from build123d import *

# Parameters (mm, degrees)
SKETCH_1_W          = 6
SKETCH_1_H          = 6
EXTRUDE_1_DEPTH     = 27
SKETCH_2_W          = 2
SKETCH_2_H          = 3
EXTRUDE_2_DEPTH     = 6
SKETCH_3_R          = 0.75
EXTRUDE_3_DEPTH     = 1
SKETCH_5_W          = 18
SKETCH_5_H          = 3.5
CUT_EXTRUDE_1_DEPTH = 8
SKETCH_6_R          = 1.5
CUT_EXTRUDE_2_DEPTH = 8
SKETCH_7_R          = 0.9
CUT_EXTRUDE_3_DEPTH = 8


with BuildPart() as part:
    # 草图1 → 凸台-拉伸1 (new body)
    with BuildSketch(Plane.XY):
        Rectangle(SKETCH_1_W, SKETCH_1_H)
    extrude(amount=EXTRUDE_1_DEPTH)

    # 草图2 → 凸台-拉伸2 (add)
    with BuildSketch(Plane.XY.offset(27)):
        with Locations((-1.14479355, -0.004540815)):
            Rectangle(SKETCH_2_W, SKETCH_2_H)
    extrude(amount=EXTRUDE_2_DEPTH)

    # 草图3 → 凸台-拉伸3 (add)
    with BuildSketch(Plane.ZY.offset(2.14479355)):
        with Locations(Location((31, 0, 0), (0, 0, 90))):
            Circle(SKETCH_3_R)
    extrude(amount=EXTRUDE_3_DEPTH)

    # 草图4 → 旋转1 (revolve)
    with BuildSketch(Plane(origin=(0, 0, 0), x_dir=(1, 0, 0), z_dir=(0, 1, 0))):
        with BuildLine():
            Line((-3.14479355, -31), (-6.998843172, -31))
            ThreePointArc((-6.998843172, -31), (-5.380877697, -29.036826645), (-3.14479355, -30.25))
            Line((-3.14479355, -30.25), (-3.14479355, -31))
        make_face()
    revolve(axis=Axis((-3.14479355, 0, 31), (-1, 0, 0)))

    # 草图5 → 切除-拉伸1 (cut)
    with BuildSketch(Plane(origin=(0.5, 3, 0), x_dir=(0, 0, 1), z_dir=(0, -1, 0))):
        with Locations((13.5, 0.5)):
            Rectangle(SKETCH_5_W, SKETCH_5_H)
    extrude(amount=CUT_EXTRUDE_1_DEPTH, mode=Mode.SUBTRACT)

    # 草图6 → 切除-拉伸2 (cut)
    with BuildSketch(Plane.ZY.offset(3)):
        with Locations((16, 0)):
            Circle(SKETCH_6_R)
    extrude(amount=-CUT_EXTRUDE_2_DEPTH, mode=Mode.SUBTRACT)

    # 草图7 → 切除-拉伸3 (cut)
    with BuildSketch(Plane(origin=(0, 0, 0), x_dir=(-1, 0, 0), z_dir=(0, 0, -1))):
        Circle(SKETCH_7_R)
    extrude(amount=-CUT_EXTRUDE_3_DEPTH, mode=Mode.SUBTRACT)


solid = part.part
Part model, mm, in its own coordinate system. A direction names the side the tool comes from. Coordinates: 2 decimals unless noted, no trailing zeros. Loops run counter-clockwise (first coordinate to the right, second up) from the corner with the lowest first, then second, coordinate; pieces in that order, holes last. Notation, with made-up numbers: M 37,-32.75 L 71,-32.75 A16 cw 71,-8.75 Z; hole C 64,80 d3. An arc over 180 degrees is marked long. Use a Markdown table: item, result. Add a question column.
Q1. Cut at A-A (y = 0). Write the cut outline in (x, z), and give its area (3 significant figures).
Q2. Mould opens along X. For faces 1 (the flat face through (-3, 0, 13)), 2 (the flat face through (-1.75, 0, 13)), 3 (the flat face through (-1, -1.505, 30)) say: +X half, -X half, draft (parallel to the pull), parting line (faces both ways), or undercut.
Q3. Cut at C-C (z = 16). Write the cut outline in (x, y), and give its area (3 significant figures).
Q4. Which spindle directions (+Z, -Z, +X, -X, +Y, -Y) get a long thin tool onto all of the face, cutting with end or side? Do faces 4 (the flat face through (-1, 1.495, 30)), 5 (the flat face through (-0.145, 0, 30)), 6 (the flat face through (1.75, 0, 13)), 7 (the cylindrical face through (-0.86, 0.27, 2.22)), 8 (the cylindrical face through (-2.638, -0.098, 30.256)). Say none if no direction does.
Q5. Pin check, flat tips, straight feed: P1, Ø3.5, axis at y = 0.5, z = 30.5, coming from the +X side; P2, Ø1.6, axis at x = -1.5, z = 30, coming from the -Y side; P3, Ø3, axis at y = 1, z = 7.5, coming from the -X side. Stop position of each tip, or through.
Q6. Cut at D-D (x = -0.5). Write the cut outline in (y, z), and give its area (3 significant figures).
Q7. Cut at B-B (x = 1.25). Write the cut outline in (y, z).
Q8. Probe L1, parallel to X at y = 2.25, z = 17; L2, parallel to Y at x = -0.5, z = 3; L3, parallel to Z at x = 1.5, y = -1. List the from-to ranges inside material, lowest first.
Worked out:
| question | item | result |
|---|---|---|
| 1 | outline | M -3.14,30.25 L -2.14,30.25 L -2.14,27 L -3,27 L -3,17.5 L -1.75,17.5 L -1.75,22.5 L 1.75,22.5 L 1.75,17.5 L 3,17.5 L 3,27 L -0.14,27 L -0.14,33 L -2.14,33 L -2.14,31.75 L -3.14,31.75 A2 ccw long Z; M -3,0 L -0.9,0 L -0.9,4.5 L -1.75,4.5 L -1.75,14.5 L -3,14.5 Z; M 0.9,0 L 3,0 L 3,14.5 L 1.75,14.5 L 1.75,4.5 L 0.9,4.5 Z |
| 1 | area | 109 mm2 |
| 2 | face 1 | -X half |
| 2 | face 2 | undercut |
| 2 | face 3 | draft |
| 3 | outline | M -3,-3 L -1.75,-3 L -1.75,-1.5 L -3,-1.5 Z; M -3,1.5 L -1.75,1.5 L -1.75,3 L -3,3 Z; M 1.75,-3 L 3,-3 L 3,-1.5 L 1.75,-1.5 Z; M 1.75,1.5 L 3,1.5 L 3,3 L 1.75,3 Z |
| 3 | area | 7.50 mm2 |
| 4 | face 4 | +Z, +X, +Y |
| 4 | face 5 | +Z, +X, +Y, -Y |
| 4 | face 6 | +Y, -Y |
| 4 | face 7 | -Z |
| 4 | face 8 | none |
| 5 | P1 | stops at x = -0.14 |
| 5 | P2 | stops at y = -1.5 |
| 5 | P3 | stops at x = -3 |
| 6 | outline | M -3,0 L -0.75,0 L -0.75,4.5 L -3,4.5 Z; M -3,22.5 L 3,22.5 L 3,27 L 1.5,27 L 1.5,33 L -1.5,33 L -1.5,27 L -3,27 Z; M 0.75,0 L 3,0 L 3,4.5 L 0.75,4.5 Z |
| 6 | area | 65.3 mm2 |
| 7 | outline | M -3,0 L 3,0 L 3,4.5 L -3,4.5 Z; M -3,22.5 L 3,22.5 L 3,27 L -3,27 Z |
| 8 | L1 | x = -3 to -1.75, 1.75 to 3 |
| 8 | L2 | y = -3 to -0.75, 0.75 to 3 |
| 8 | L3 | z = 0 to 4.5, 22.5 to 27 |
